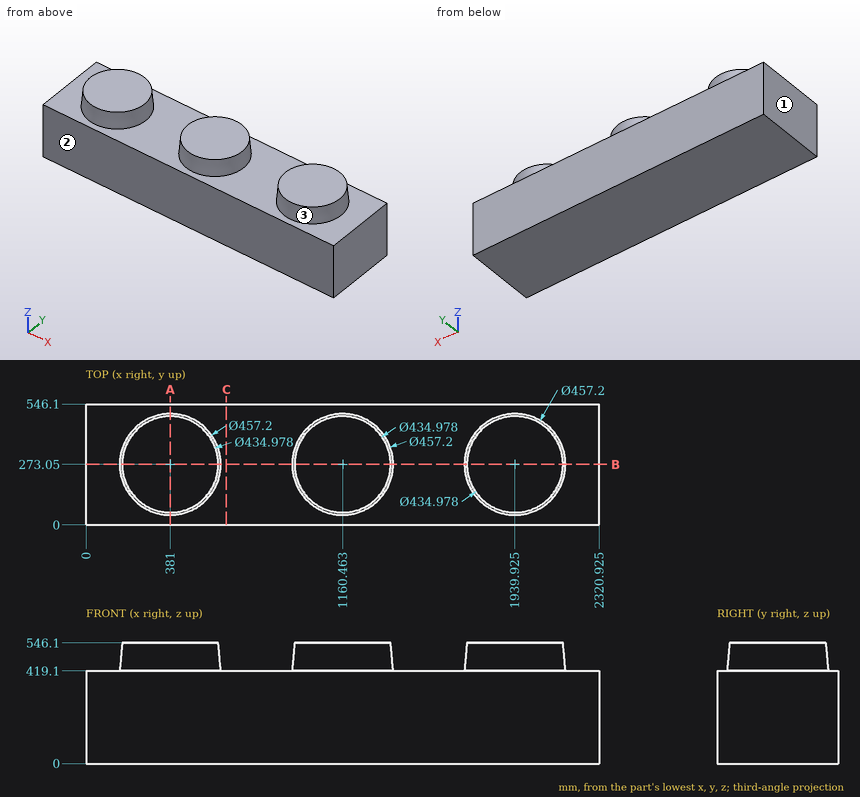
The figure shows three views and two pictorial views of one solid part (mm, origin at its lowest corner). Answer the questions. Coordinates: 2 decimals unless noted, no trailing zeros. Order: outer loops, then holes, each group sorted by start corner. A loop starts at its lowest first (then second) coordinate and runs counter-clockwise, first axis right, second up. Notation, with made-up numbers: (-14.5, -6) - (33.5, -6) arc R25 ccw to (33.5, 8) - close; hole circle Ø11 at (10.5, 45). An arc over 180 degrees is marked (long way). Answer as a JSON object with one key per item and string values.
1. Each of these flat-tipped pins is pushed along its axis until it touches: P1, Ø3, axis at x = 644.5, y = 199.5, coming from the +Z side; P2, Ø12, axis at y = 367, z = 441, coming from the -X side. Where does it stop, or does it pass through?
Output values:
{"P1": "stops at z = 419.1", "P2": "stops at x = 172.01"}
2. The mould has two halves that part along X. Classify the marked faces 1, 2 and 3: +X half, -X half, draft (parallel to the pull), parting line (faces both ways), or undercut.
Output values:
{"face 1": "-X half", "face 2": "draft", "face 3": "undercut"}
3. Find section C-C on x = 634.5. Determine the outline of the cut face in (y, z).
Output values:
{"outline": "(0, 0) - (546.1, 0) - (546.1, 419.1) - (0, 419.1) - close"}
4. Consider line 1 (Z direction, x = 1572, y = 25.5); line 2 (X direction, y = 435.5, z = 491) (1 decimal); line 3 (Y direction, x = 2000, z = 506.5). Determine where each line is inside the solid, lowest interval first.
Output values:
{"line 1": "z = 0 to 419.1", "line 2": "x = 229.2 to 532.8, 1008.7 to 1312.2, 1788.2 to 2091.7", "line 3": "y = 60.42 to 485.68"}
5. Find section B-B on y = 273.05. Determine the outline of the cut face in (x, z) (1 decimal).
Output values:
{"outline": "(0, 0) - (2320.9, 0) - (2320.9, 419.1) - (2168.5, 419.1) - (2157.4, 546.1) - (1722.4, 546.1) - (1711.3, 419.1) - (1389.1, 419.1) - (1378, 546.1) - (943, 546.1) - (931.9, 419.1) - (609.6, 419.1) - (598.5, 546.1) - (163.5, 546.1) - (152.4, 419.1) - (0, 419.1) - close"}
6. Find section A-A on x = 381. Determine the outline of the cut face in (y, z), plus the area to 3 significant figures.
Output values:
{"outline": "(0, 0) - (546.1, 0) - (546.1, 419.1) - (501.65, 419.1) - (490.54, 546.1) - (55.56, 546.1) - (44.45, 419.1) - (0, 419.1) - close", "area": "286,000 mm²"}
